```python
from build123d import *

# Parameters (mm, degrees)
SKETCH1_W                    = 15.875
SKETCH1_H                    = 9.525
BOSS_EXTRUDE1_DEPTH          = 7.9375
BOSS_EXTRUDE2_DEPTH          = 22.225
F_3_8_0_375_DIAMETER_HOLE1_D = 9.525
F_6_32_TAPPED_HOLE1_D        = 2.7051
F_8_CLEARANCE_HOLE1_D        = 4.4958
F_8_CLEARANCE_HOLE1_DEPTH    = 19.05
F_8_CLEARANCE_HOLE1_TIP      = 1.350674586


with BuildPart() as part:
    # Sketch1 → Boss-Extrude1 (new body, symmetric)
    with BuildSketch(Plane(origin=(0, 0, 0), x_dir=(0, 0, -1), z_dir=(1, 0, 0))):
        Rectangle(SKETCH1_W, SKETCH1_H)
    extrude(amount=BOSS_EXTRUDE1_DEPTH, both=True)

    # Sketch2 → Boss-Extrude2 (add)
    with BuildSketch(Plane(origin=(7.9375, 0, 0), x_dir=(0, 0, -1), z_dir=(1, 0, 0))):
        Polygon((-6.749941848, -0.656609937), (5.517316146, -3.94361181), (6.749941848, 0.656609937), (-5.517316146, 3.94361181), align=None)
    extrude(amount=BOSS_EXTRUDE2_DEPTH)

    # 3/8 (0.375) Diameter Hole1 (through all)
    with Locations(Plane(origin=(0, 4.7625, 0), x_dir=(1, 0, 0), z_dir=(0, 1, 0))):
        with Locations((0, 0)):
            Hole(F_3_8_0_375_DIAMETER_HOLE1_D / 2)

    # #6-32 Tapped Hole1 (through all)
    with Locations(Plane(origin=(0, 2.300110874, -0.616312851), x_dir=(1, 0, 0), z_dir=(0, 0.965925826, -0.258819045))):
        with Locations((24, 0)):
            Hole(F_6_32_TAPPED_HOLE1_D / 2)

    # #8 Clearance Hole1
    with Locations(Plane(origin=(-7.9375, 0, 0), x_dir=(0, 0, -1), z_dir=(-1, 0, 0))):
        with Locations((0, 0)):
            Hole(F_8_CLEARANCE_HOLE1_D / 2, depth=F_8_CLEARANCE_HOLE1_DEPTH)
            with Locations((0, 0, -(F_8_CLEARANCE_HOLE1_DEPTH + F_8_CLEARANCE_HOLE1_TIP / 2))):  # 118° drill point
                Cone(0, F_8_CLEARANCE_HOLE1_D / 2, F_8_CLEARANCE_HOLE1_TIP, mode=Mode.SUBTRACT)


solid = part.part
```
The listing builds one solid part. Answer for the finished solid, in the listing's coordinates (mm). A direction names the side the tool comes from. Give positions to 0.01 mm unless a question says otherwise; leave off trailing zeros. Write each loop counter-clockwise with the first axis right and the second up, starting at its lowest first coordinate (ties: lowest second). Pieces come first, ordered by that corner, then holes. Notation, with made-up numbers: M -40,78 L -8,78 A34 cw -8,116 Z; hole C -7.75,-19 d4. An arc over 180 degrees is marked long. Write each question's results on one line, items separated by ' | '.
Q1. For a pull along Y with two mould halves and no side action, classify faces 6 (the flat face through (-7.938, 2, 2)), 7 (the flat face through (4, 4.762, -3)), 8 (the cylindrical face through (7.7, -2.23, -0.29)) as released by +Y, released by -Y, zero draft, split by the parting line, or undercut.
Output values:
face 6: zero draft | face 7: released by +Y | face 8: undercut
Q2. Flat-ended cylindrical pins translate along their axes: P1, Ø1, axis at y = -1.5, z = 4, coming from the +X side; P2, Ø1.5, axis at x = 9, y = -0.5, coming from the -Z side; P3, Ø5, axis at x = 13, y = 2, coming from the +Z side. Find the tip coordinate at first contact, or state that the pin passes through.
Output values:
P1: x = 30.16 | P2: z = -6.64 | P3: z = 6.71
Q3. Section D-D, the plane y = -3.5 is taken. Write down the section's boundary in (x, z) (1 decimal), then the cut area to 3 significant figures.
Output values:
outline: M -7.9,-7.9 L 7.9,-7.9 L 7.9,-5.6 L 30.2,-5.6 L 30.2,-3.9 L 7.9,-3.9 L 7.9,7.9 L -7.9,7.9 Z; hole C 0,0 d9.5 | area: 220 mm2
Q4. Section B-B, the plane z = -4.25 is taken. Write down the section's boundary in (x, y), then the cut area to 3 significant figures.
Output values:
outline: M -7.94,-4.76 L -2.15,-4.76 L -2.15,4.76 L -7.94,4.76 Z; M 2.15,-4.76 L 7.94,-4.76 L 7.94,-3.6 L 30.16,-3.6 L 30.16,1.33 L 7.94,1.33 L 7.94,4.76 L 2.15,4.76 Z | area: 220 mm2
Q5. Section A-A, the plane x = 0 is taken. Write down the section's boundary in (y, z), then the cut area to 3 significant figures.
Output values:
outline: M -4.76,-7.94 L 4.76,-7.94 L 4.76,-4.76 L -4.76,-4.76 Z; M -4.76,4.76 L 4.76,4.76 L 4.76,7.94 L -4.76,7.94 Z | area: 60.5 mm2
Q6. A tool of negligible diameter and unlimited length cuts with its end or side. For faces 1 (the flat face through (18.894, 1.676, 6.125)), 2 (the cylindrical face through (-6.042, 0.861, 2.076)), 3 (the flat face through (18.894, -2.277, 0.702)), 4 (the flat face through (18.894, -1.676, -6.125)), 5 (the flat face through (18.894, 2.277, -0.702)), from which of +Z, -Z, +X, -X, +Y, -Y can it reach the whole face along a straight path? Write none if from no direction.
Output values:
face 1: +Z, +X, +Y | face 2: -X | face 3: +Z, +X, -Y | face 4: -Z, +X, -Y | face 5: -Z, +X, +Y
Q7. Section C-C, the plane x = 10.5 is taken. Write down the section's boundary in (y, z).
Output values:
outline: M -3.94,-5.52 L 0.66,-6.75 L 3.94,5.52 L -0.66,6.75 Z; hole C 0,0 d4.5
Q8. Consider L1, parallel to Y at x = -6.3, z = 0; L2, parallel to Z at x = 0, y = -1; L3, parallel to Y at x = 9.5, z = 0. Determine where each line is inside the solid, lowest interval first. Write a range as from..to.
Output values:
L1: -4.76..-2.25, 2.25..4.76 | L2: -7.94..-4.76, 4.76..7.94 | L3: -2.47..-2.25, 2.25..2.47
